Source: CAD feature listing. Evaluate the final solid. Frame: model axes, mm. Face numbers are marked on the shaded views. A direction names the side the tool comes from. Coordinates: 2 decimals unless noted, no trailing zeros. Write each loop counter-clockwise with the first axis right and the second up, starting at its lowest first coordinate (ties: lowest second). Pieces come first, ordered by that corner, then holes. Notation, with made-up numbers: (19.25, -39) - (30.25, -39) arc R13 cw to (30.25, -24) - close; hole circle Ø5 at (-25.5, -36.75). An arc over 180 degrees is marked (long way). One line per item, written item: value.
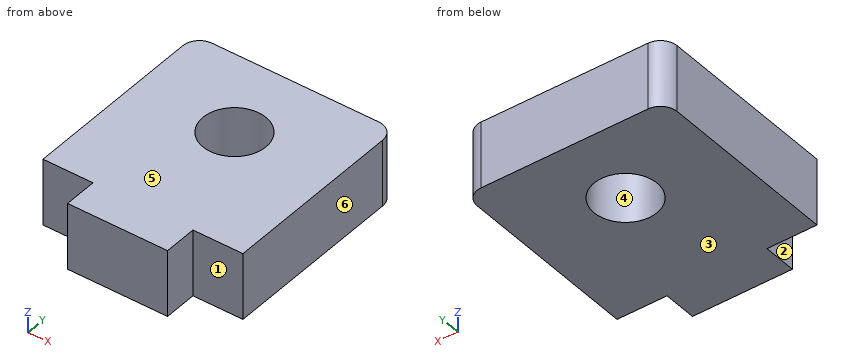
from build123d import *

# Parameters (mm, degrees)
SKETCH1_R           = 3
SKETCH1_W           = 9.525
SKETCH1_H           = 3.175
BOSS_EXTRUDE1_DEPTH = 6.35
FILLET1_R           = 1.5875


with BuildPart() as part:
    # Sketch1 → Boss-Extrude1 (new body)
    # profile 1 of 2: a face of its own
    with BuildSketch(Plane.XY):
        Polygon((9.525, 11.1125), (-9.525, 11.1125), (-9.525, -7.9375), (-4.7625, -7.9375), (4.7625, -7.9375), (9.525, -7.9375), align=None)
        with Locations((0, 3.4925)):
            Circle(SKETCH1_R, mode=Mode.SUBTRACT)
    # profile 2 of 2: a face of its own
    with BuildSketch(Plane.XY):
        with Locations((0, -9.525)):
            Rectangle(SKETCH1_W, SKETCH1_H)
    extrude(amount=BOSS_EXTRUDE1_DEPTH)

    # Fillet1
    fillet1_edges = [part.edges().sort_by_distance(p)[0] for p in [
        (-9.525, 11.1125, 3.175),
        (9.525, 11.1125, 3.175),
    ]]
    fillet(fillet1_edges, radius=FILLET1_R)


solid = part.part
1) Section query D-D on x = -5.25. Output: boundary loops of the cut face in (y, z).
Values found:
outline: (-7.94, 0) - (11.11, 0) - (11.11, 6.35) - (-7.94, 6.35) - close
2) Material intervals for line 1 (Y direction, x = 0, z = 4); line 2 (X direction, y = 3.5, z = 4.75) (3 decimals); line 3 (Y direction, x = 6.5, z = 2.5), sorted ascending.
Values found:
line 1: -11.11 to 0.49, 6.49 to 11.11
line 2: -9.525 to -3, 3 to 9.525
line 3: -7.94 to 11.11
3) Section query B-B on z = 5.5. Output: boundary loops of the cut face in (x, y) (1 decimal), then the cut area to 3 significant figures.
Values found:
outline: (-9.5, -7.9) - (-4.8, -7.9) - (-4.8, -11.1) - (4.8, -11.1) - (4.8, -7.9) - (9.5, -7.9) - (9.5, 9.5) arc R1.6 ccw to (7.9, 11.1) - (-7.9, 11.1) arc R1.6 ccw to (-9.5, 9.5) - close; hole circle Ø6 at (0, 3.5)
area: 364 mm2
4) Reachability of the marked faces 1, 2 and 3 from +Z, -Z, +X, -X, +Y, -Y: full face, straight path, thin tool, end or side. Return the list, or none.
Values found:
face 1: +Z, -Z, +X, -Y
face 2: +Z, -Z, -X, -Y
face 3: -Z, +X, -X, +Y, -Y
5) Section query C-C on y = -9.25. Output: boundary loops of the cut face in (x, z).
Values found:
outline: (-4.76, 0) - (4.76, 0) - (4.76, 6.35) - (-4.76, 6.35) - close
6) Section query A-A on x = 0. Output: boundary loops of the cut face in (y, z), then the cut area to 3 significant figures.
Values found:
outline: (-11.11, 0) - (0.49, 0) - (0.49, 6.35) - (-11.11, 6.35) - close; (6.49, 0) - (11.11, 0) - (11.11, 6.35) - (6.49, 6.35) - close
area: 103 mm2
7) Contact query for flat-ended pins moving along their axis: P1, Ø1, axis at y = -9.5, z = 1.5, coming from the -X side; P2, Ø1.4, axis at x = 6.5, z = 4.5, coming from the -Y side. Output: stop coordinate, or through.
Values found:
P1: x = -4.76
P2: y = -7.94
8) Draft query along X for the marked faces 4, 5 and 6. Return one class per face: released by +X, released by -X, zero draft, split by the parting line, or undercut.
Values found:
face 4: undercut
face 5: zero draft
face 6: released by +X
